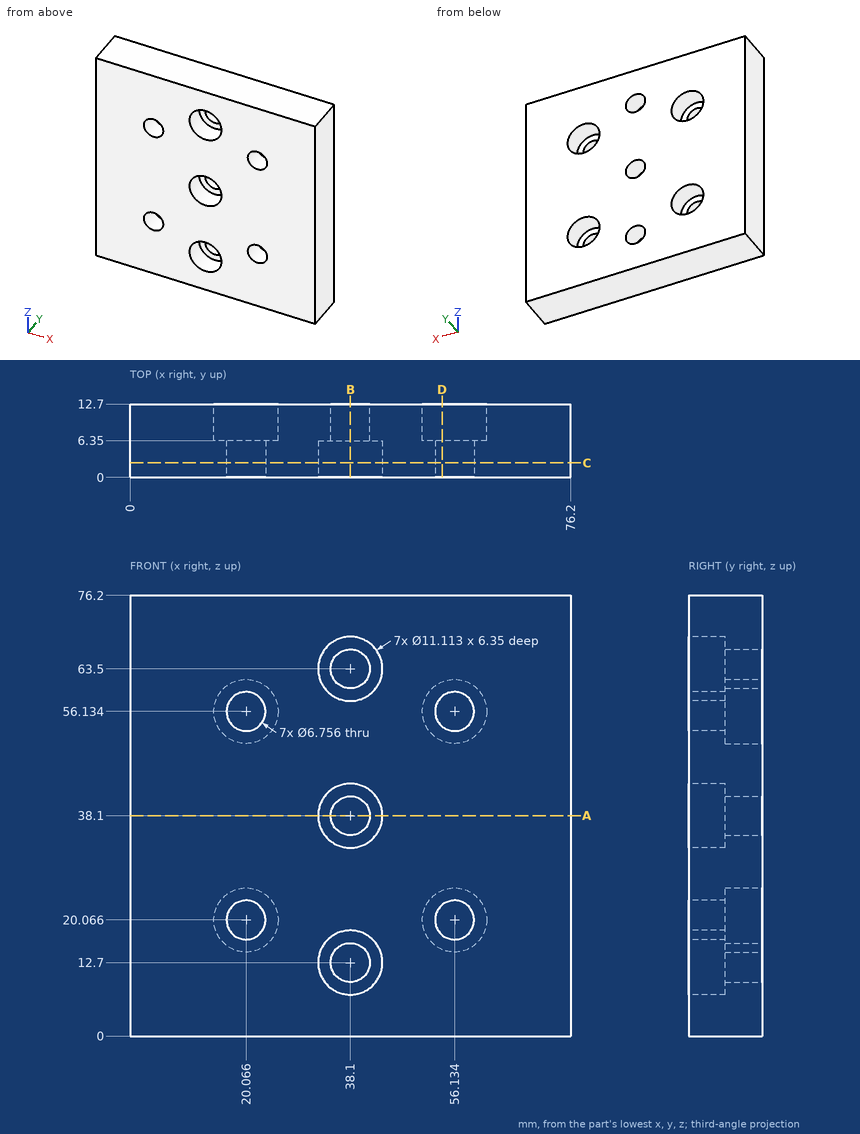
Geometry: see drawing. Coordinates: mm, zero at the bounding-box minimum. Round coordinates to 2 decimals unless told otherwise and drop trailing zeros. Loops run counter-clockwise (first coordinate to the right, second up) from the corner with the lowest first, then second, coordinate; pieces in that order, holes last. Notation, with made-up numbers: M 21.5,29.5 L 47.5,29.5 A22 cw 47.5,48.5 Z; hole C 41.25,-35.75 d10. An arc over 180 degrees is marked long. Use a Markdown table: item, result. Add a question column.
1. Cut plane B-B, the plane x = 38.1. Output: boundary loops of the cut face in (y, z).
2. Cut plane D-D, the plane x = 54. State how many separate pieces and enclosed holes the cut face has, and give its area (3 significant figures).
3. Ray query, line 1 along Z through (x, y) = (38.1, 4.75); line 2 along Z through (x, y) = (38.1, 9); line 3 along X through (y, z) = (5.5, 63.5). Return the intervals inside material, ascending. Write a range as [from, to].
4. Cut plane C-C, the plane y = 2.5. Output: boundary loops of the cut face in (x, z) (1 decimal).
5. Cut plane A-A, the plane z = 38.1. Output: boundary loops of the cut face in (x, y), and give its area (3 significant figures).
6. Contact query for flat-ended pins moving along their axis: pin 1 (8 mm diameter, centred on x = 20.066, z = 56.134, fed in from +Y); pin 2 (6.5 mm diameter, centred on x = 20.066, z = 20.066, fed in from -Y); pin 3 (9 mm diameter, centred on x = 38.1, z = 12.7, fed in from -Y). Output: stop coordinate, or through.
Solution:
| question | item | result |
|---|---|---|
| 1 | outline | M 0,0 L 12.7,0 L 12.7,9.32 L 6.35,9.32 L 6.35,7.14 L 0,7.14 Z; M 0,18.26 L 6.35,18.26 L 6.35,16.08 L 12.7,16.08 L 12.7,34.72 L 6.35,34.72 L 6.35,32.54 L 0,32.54 Z; M 0,43.66 L 6.35,43.66 L 6.35,41.48 L 12.7,41.48 L 12.7,60.12 L 6.35,60.12 L 6.35,57.94 L 0,57.94 Z; M 0,69.06 L 6.35,69.06 L 6.35,66.88 L 12.7,66.88 L 12.7,76.2 L 0,76.2 Z |
| 2 | separate pieces | 3 |
| 2 | enclosed holes | 0 |
| 2 | area | 771 mm2 |
| 3 | line 1 | z = [0, 7.14], [18.26, 32.54], [43.66, 57.94], [69.06, 76.2] |
| 3 | line 2 | z = [0, 9.32], [16.08, 34.72], [41.48, 60.12], [66.88, 76.2] |
| 3 | line 3 | x = [0, 32.54], [43.66, 76.2] |
| 4 | outline | M 0,0 L 76.2,0 L 76.2,76.2 L 0,76.2 Z; hole C 20.1,20.1 d6.8; hole C 20.1,56.1 d6.8; hole C 38.1,12.7 d11.1; hole C 38.1,38.1 d11.1; hole C 38.1,63.5 d11.1; hole C 56.1,20.1 d6.8; hole C 56.1,56.1 d6.8 |
| 5 | outline | M 0,0 L 32.54,0 L 32.54,6.35 L 34.72,6.35 L 34.72,12.7 L 0,12.7 Z; M 41.48,6.35 L 43.66,6.35 L 43.66,0 L 76.2,0 L 76.2,12.7 L 41.48,12.7 Z |
| 5 | area | 854 mm2 |
| 6 | pin 1 | stops at y = 6.35 |
| 6 | pin 2 | passes through |
| 6 | pin 3 | stops at y = 6.35 |
